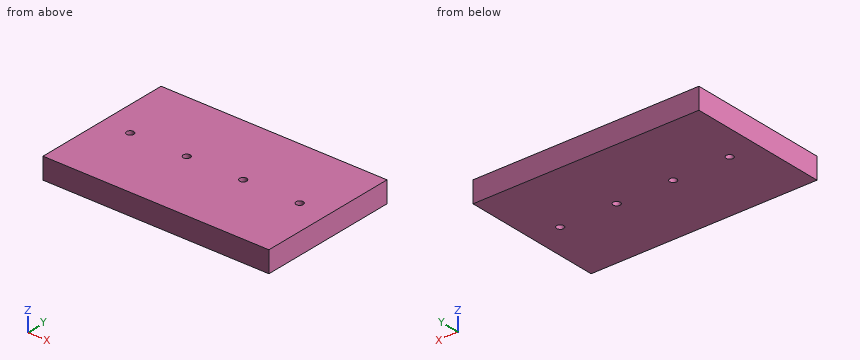
Autodesk Inventor part; units mm, degrees
ref_plane "YZ Plane" through (0, 0, 0) normal (1, 0, 0) x (0, 1, 0)
ref_plane "XZ Plane" through (0, 0, 0) normal (0, 1, 0) x (-1, 0, 0)
ref_plane "XY Plane" through (0, 0, 0) normal (0, 0, 1) x (1, 0, 0)
sketch "Sketch1" plane through (0, 0, 0) normal (0, 0, 1) x (1, 0, 0)
  line L0 (-101.6, 63.5) -> (101.6, 63.5)
  line L1 (101.6, 63.5) -> (101.6, -63.5)
  line L2 (101.6, -63.5) -> (-101.6, -63.5)
  line L3 (-101.6, -63.5) -> (-101.6, 63.5)
  line L4 (-101.6, 63.5) -> (101.6, -63.5) construction
  line L5 (101.6, 63.5) -> (-101.6, -63.5) construction
  circle A0 centre (-76.2, 0) radius 3.175
  circle A1 centre (-25.4, 0) radius 3.175
  circle A2 centre (25.4, 0) radius 3.175
  circle A3 centre (76.2, 0) radius 3.175
  point P0 (0, 0)
  dimension "d0" = 203.2
  dimension "d1" = 127
  dimension "d2" = 6.35
  dimension "d3" = 6.35
  dimension "d4" = 6.35
  dimension "d5" = 6.35
  dimension "d6" = 25.4
  dimension "d7" = 76.2
  dimension "d8" = 127
  dimension "d9" = 177.8
extrude "Extrusion1" add sketch "Sketch1" along normal blind 19.05 contours L0 L1 L2 L3 | A0 | A1 | A2 | A3
sketch "Sketch2" plane through (0, 0, 0) normal (0, 0, -1) x (-1, 0, 0)
  circle A0 centre (-76.2, 0) radius 3.175
  circle A1 centre (-25.4, 0) radius 3.175
  circle A2 centre (25.4, 0) radius 3.175
  circle A3 centre (76.2, 0) radius 3.175
  line L0 (-101.6, 63.5) -> (101.6, 63.5)
  line L1 (-101.6, -63.5) -> (-101.6, 63.5)
  point P0 (0, 0)
  dimension "d12" = 6.35
  dimension "d13" = 6.35
  dimension "d14" = 6.35
  dimension "d15" = 6.35
  dimension "d17" = 63.5
  dimension "d18" = 63.5
  dimension "d19" = 25.4
  dimension "d20" = 76.2
  dimension "d21" = 127
  dimension "d22" = 177.8
extrude "Extrusion2" cut sketch "Sketch2" against normal blind 19.05
properties part number "Part_Back"
The listing builds one solid part. Answer for the finished solid, in the listing's coordinates (mm). Coordinates: 2 decimals unless noted, no trailing zeros. Loops run counter-clockwise (first coordinate to the right, second up) from the corner with the lowest first, then second, coordinate; pieces in that order, holes last. Notation, with made-up numbers: M 26.25,60 L 76.25,60 A31 cw 76.25,92 Z; hole C -8.75,12.5 d2. An arc over 180 degrees is marked long. Answer as a JSON object with one key per item and string values. Group by question number.
Item 1: Section A-A (y = 0) is taken. Write down the section's boundary in (x, z) (3 decimals), and give its area (3 significant figures).
Item 2: Section B-B (x = 25.4) is taken. Write down the section's boundary in (y, z) (3 decimals).
Item 3: Consider L1, parallel to Y at x = -76.2, z = 13 (3 decimals); L2, parallel to Y at x = -78.5, z = 1.75. Determine where each line is inside the solid, lowest interval first.
Solved:
{
 "1": {"outline": "M -101.6,0 L -79.375,0 L -79.375,19.05 L -101.6,19.05 Z; M -73.025,0 L -28.575,0 L -28.575,19.05 L -73.025,19.05 Z; M -22.225,0 L 22.225,0 L 22.225,19.05 L -22.225,19.05 Z; M 28.575,0 L 73.025,0 L 73.025,19.05 L 28.575,19.05 Z; M 79.375,0 L 101.6,0 L 101.6,19.05 L 79.375,19.05 Z", "area": "3,390 mm2"},
 "2": {"outline": "M -63.5,0 L -3.175,0 L -3.175,19.05 L -63.5,19.05 Z; M 3.175,0 L 63.5,0 L 63.5,19.05 L 3.175,19.05 Z"},
 "3": {"L1": "y = -63.5 to -3.175, 3.175 to 63.5", "L2": "y = -63.5 to -2.19, 2.19 to 63.5"}
}
